from build123d import *

# Parameters (mm, degrees)
ESQUISSE1_W         = 30.8
ESQUISSE1_H         = 30.8
BOSS_EXTRU_1_DEPTH  = 15
ESQUISSE6_W         = 155.98
ESQUISSE6_H         = 200
BOSS_EXTRU_4_DEPTH  = 10
ESQUISSE16_W        = 30.8
ESQUISSE16_H        = 30.8
BOSS_EXTRU_12_DEPTH = 15
ESQUISSE25_W        = 30.8
ESQUISSE25_H        = 30.8
BOSS_EXTRU_21_DEPTH = 15
ESQUISSE26_W        = 30.8
ESQUISSE26_H        = 30.8
BOSS_EXTRU_22_DEPTH = 15


with BuildPart() as part:
    # Esquisse1 → Boss.-Extru.1 (new body)
    with BuildSketch(Plane.XY):
        with Locations((-26.267627057, 8.434243976)):
            Rectangle(ESQUISSE1_W, ESQUISSE1_H)
        Polygon((-30.117627057, 6.034243976), (-30.117627057, 10.834243976), (-36.367627057, 10.834243976), (-36.367627057, 18.534243976), (-28.667627057, 18.534243976), (-28.667627057, 12.284243976), (-23.867627057, 12.284243976), (-23.867627057, 18.534243976), (-16.177627057, 18.534243976), (-16.177627057, 10.834243976), (-22.427627057, 10.834243976), (-22.427627057, 6.034243976), (-16.177627057, 6.034243976), (-16.177627057, -1.665756024), (-23.867627057, -1.665756024), (-23.867627057, 4.584243976), (-28.667627057, 4.584243976), (-28.667627057, -1.665756024), (-36.367627057, -1.665756024), (-36.367627057, 6.034243976), align=None, mode=Mode.SUBTRACT)
    extrude(amount=BOSS_EXTRU_1_DEPTH)

    # Esquisse6 → Boss.-Extru.4 (add)
    with BuildSketch(Plane(origin=(0, 23.834243976, 0), x_dir=(1, 0, 0), z_dir=(0, 1, 0))):
        with Locations((36.322372943, 85)):
            Rectangle(ESQUISSE6_W, ESQUISSE6_H)
    extrude(amount=BOSS_EXTRU_4_DEPTH)

    # Esquisse16 → Boss.-Extru.12 (add)
    with BuildSketch(Plane.XY.offset(15)):
        with Locations((98.912372943, 8.434243976)):
            Rectangle(ESQUISSE16_W, ESQUISSE16_H)
        Polygon((95.062372943, 6.034243976), (95.062372943, 10.834243976), (88.812372943, 10.834243976), (88.812372943, 18.534243976), (96.512372943, 18.534243976), (96.512372943, 12.284243976), (101.312372943, 12.284243976), (101.312372943, 18.534243976), (109.002372943, 18.534243976), (109.002372943, 10.834243976), (102.752372943, 10.834243976), (102.752372943, 6.034243976), (109.002372943, 6.034243976), (109.002372943, -1.665756024), (101.312372943, -1.665756024), (101.312372943, 4.584243976), (96.512372943, 4.584243976), (96.512372943, -1.665756024), (88.812372943, -1.665756024), (88.812372943, 6.034243976), align=None, mode=Mode.SUBTRACT)
    extrude(amount=-BOSS_EXTRU_12_DEPTH)

    # Esquisse25 → Boss.-Extru.21 (add)
    with BuildSketch(Plane(origin=(0, 0, -185), x_dir=(-1, 0, 0), z_dir=(0, 0, -1))):
        with Locations((-98.912372943, 8.434243976)):
            Rectangle(ESQUISSE25_W, ESQUISSE25_H)
        Polygon((-102.762372943, 6.034243976), (-102.762372943, 10.834243976), (-109.012372943, 10.834243976), (-109.012372943, 18.534243976), (-101.312372943, 18.534243976), (-101.312372943, 12.284243976), (-96.512372943, 12.284243976), (-96.512372943, 18.534243976), (-88.822372943, 18.534243976), (-88.822372943, 10.834243976), (-95.072372943, 10.834243976), (-95.072372943, 6.034243976), (-88.822372943, 6.034243976), (-88.822372943, -1.665756024), (-96.512372943, -1.665756024), (-96.512372943, 4.584243976), (-101.312372943, 4.584243976), (-101.312372943, -1.665756024), (-109.012372943, -1.665756024), (-109.012372943, 6.034243976), align=None, mode=Mode.SUBTRACT)
    extrude(amount=-BOSS_EXTRU_21_DEPTH)

    # Esquisse26 → Boss.-Extru.22 (add)
    with BuildSketch(Plane(origin=(0, 0, -185), x_dir=(-1, 0, 0), z_dir=(0, 0, -1))):
        with Locations((26.267627057, 8.434243976)):
            Rectangle(ESQUISSE26_W, ESQUISSE26_H)
        Polygon((22.417627057, 6.034243976), (22.417627057, 10.834243976), (16.167627057, 10.834243976), (16.167627057, 18.534243976), (23.867627057, 18.534243976), (23.867627057, 12.284243976), (28.667627057, 12.284243976), (28.667627057, 18.534243976), (36.357627057, 18.534243976), (36.357627057, 10.834243976), (30.107627057, 10.834243976), (30.107627057, 6.034243976), (36.357627057, 6.034243976), (36.357627057, -1.665756024), (28.667627057, -1.665756024), (28.667627057, 4.584243976), (23.867627057, 4.584243976), (23.867627057, -1.665756024), (16.167627057, -1.665756024), (16.167627057, 6.034243976), align=None, mode=Mode.SUBTRACT)
    extrude(amount=-BOSS_EXTRU_22_DEPTH)


solid = part.part
Geometry check sheet. Reference: the model listing, model coordinates, mm. A direction names the side the tool comes from. Round coordinates to 2 decimals unless told otherwise and drop trailing zeros. Write each loop counter-clockwise with the first axis right and the second up, starting at its lowest first coordinate (ties: lowest second). Pieces come first, ordered by that corner, then holes. Notation, with made-up numbers: (-16.5, 32) -> (7.5, 32) arc R13 ccw to (7.5, 56) -> close; hole circle Ø4 at (-38, 86.25). An arc over 180 degrees is marked (long way). One line per item, written item: value. Start each with the question number.
(1) Cross-section at A-A, the plane y = 1. Give the number of separate pieces and of enclosed holes in the cut face, and give its area (3 significant figures).
(2) Access from +Z, -Z, +X, -X, +Y, -Y to the whole of each face (thin tool, end or side, straight path). Record for faces 1 (the flat face through (-20, 18.534, 7)), 2 (the flat face through (-10.868, 8, -178)).
(3) Cross-section at B-B, the plane z = -34. Record the cut outline in (x, y).
(4) Go/stop test with a flat-tipped pin: pin 1 Ø3 at (x, z) = (5, -36.5) entering from -Y. Record where the tip stops, or that it passes through.
(5) Scan lines: line 1 (Z direction, x = -24.5, y = -0.5); line 2 (Y direction, x = 6, z = 7.5). Record each from-to range of solid material in increasing order. Write a range as [from, to].
(6) Cross-section at C-C, the plane x = 53. Record the cut outline in (y, z), and give its area (3 significant figures).
Answer:
1. separate pieces: 12
1. enclosed holes: 0
1. area: 925 mm²
2. face 1: +Z, -Z
2. face 2: +Z, -Z, -Y
3. outline: (-41.67, 23.83) -> (114.31, 23.83) -> (114.31, 33.83) -> (-41.67, 33.83) -> close
4. pin 1: y = 23.83
5. line 1: [-185, -170], [0, 15]
5. line 2: [23.83, 33.83]
6. outline: (23.83, -185) -> (33.83, -185) -> (33.83, 15) -> (23.83, 15) -> close
6. area: 2,000 mm²
